Design review of the part built by this model. Coordinates are the model's own, in mm. Face numbers are marked on the shaded views. Coordinates: 2 decimals unless noted, no trailing zeros. Loops run counter-clockwise (first coordinate to the right, second up) from the corner with the lowest first, then second, coordinate; pieces in that order, holes last. Notation, with made-up numbers: M 56.25,8 L 91.25,8 A25 cw 91.25,43 Z; hole C 18.25,60.5 d5. An arc over 180 degrees is marked long. One line per item, written item: value.
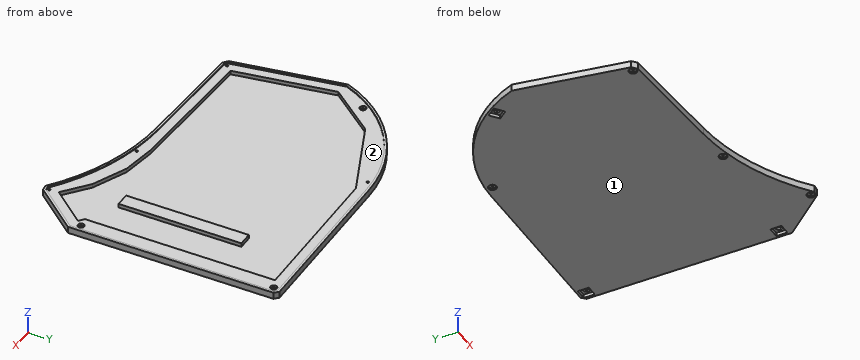
```python
from build123d import *

# Parameters (mm, degrees)
PAD001_DEPTH         = 3.4
POCKET006_DEPTH      = 0.4
SKETCH011_R          = 1.6
SKETCH011_W          = 7
SKETCH011_H          = 62
POCKET007_DEPTH      = 2
SKETCH012_W          = 5.6
SKETCH012_H          = 5.6
POCKET008_DEPTH      = 1.8
SKETCH014_R          = 0.6
POCKET010_DEPTH      = 0.001
POCKET010_DEPTH_BACK = 3.401
SKETCH016_R          = 2
POCKET012_DEPTH      = 1


with BuildPart() as part:
    # Sketch009 → Pad001 (new body)
    with BuildSketch(Plane(origin=(-70.9, 59.5, 0), x_dir=(1, 0, 0), z_dir=(0, 0, 1))):
        with BuildLine():
            ThreePointArc((129.954505, -55.0425), (90.803609, -67.301419), (65.635795, -99.699797))
            Line((65.635795, -99.699797), (75.365663, -154.835718))
            Line((75.365663, -154.835718), (77.709881, -156.921033))
            Line((77.709881, -156.921033), (133.968943, -160.182427))
            ThreePointArc((195.00443, -183.822904), (166.343475, -167.208769), (133.968943, -160.182427))
            Line((195.00443, -183.822904), (197.834526, -183.566965))
            Line((197.834526, -183.566965), (216.95, -160.867339))
            Line((216.95, -160.867339), (216.95, -57.0425))
            Line((214.95, -55.0425), (216.95, -57.0425))
            Line((214.95, -55.0425), (129.954505, -55.0425))
        make_face()
    extrude(amount=PAD001_DEPTH)

    # Sketch010 → Pocket006 (cut)
    with BuildSketch(Plane(origin=(-70.9, 59.5, 3.4), x_dir=(1, 0, 0), z_dir=(0, 0, 1))):
        with BuildLine():
            ThreePointArc((129.954505, -56.2425), (91.621754, -68.194493), (66.874586, -99.814544))
            Line((66.874586, -99.814544), (76.474909, -154.216377))
            Line((76.474909, -154.216377), (78.195777, -155.747186))
            Line((78.195777, -155.747186), (134.038391, -158.984439))
            ThreePointArc((195.379997, -182.584043), (166.5491, -166.00184), (134.038391, -158.984439))
            Line((195.379997, -182.584043), (197.234685, -182.416314))
            Line((197.234685, -182.416314), (215.75, -160.429378))
            Line((215.75, -160.429378), (215.75, -57.539556))
            Line((215.75, -57.539556), (214.452944, -56.2425))
            Line((214.452944, -56.2425), (129.954505, -56.2425))
        make_face()
    extrude(amount=-POCKET006_DEPTH, mode=Mode.SUBTRACT)

    # Sketch011 → Pocket007 (cut)
    with BuildSketch(Plane(origin=(-70.9, 59.5, 3), x_dir=(1, 0, 0), z_dir=(0, 0, 1))):
        with Locations((212.95, -59.0425)):
            Circle(SKETCH011_R)
        with Locations((212.95, -156.302532)):
            Circle(SKETCH011_R)
        with Locations((77.4441, -85.981596)):
            Circle(SKETCH011_R)
        Polygon((72.012841, -101.311041), (90.572874, -77.866788), (131.149099, -61.0425), (207.95, -61.0425), (207.95, -87.0425), (207.95, -156.967837), (210.542474, -159.161469), (195.830749, -176.631643), (183.495202, -166.193872), (166.255124, -158.080894), (149.066225, -155.047559), (80.797353, -151.089943), align=None)
        with Locations((187.45, -118.0425)):
            Rectangle(SKETCH011_W, SKETCH011_H, mode=Mode.SUBTRACT)
    extrude(amount=-POCKET007_DEPTH, mode=Mode.SUBTRACT)

    # Sketch012 → Pocket008 (cut)
    with BuildSketch(Plane(origin=(-70.9, 59.5, 0), x_dir=(1, 0, 0), z_dir=(0, 0, 1))):
        Polygon((81.377006, -85.514821), (76.978793, -82.04845), (73.512422, -86.446662), (77.910635, -89.913033), align=None)
        with Locations((212.95, -59.0425)):
            Rectangle(SKETCH012_W, SKETCH012_H)
        with Locations((212.95, -156.302532)):
            Rectangle(SKETCH012_W, SKETCH012_H)
    extrude(amount=POCKET008_DEPTH, mode=Mode.SUBTRACT)

    # Sketch014 → Pocket010 (cut, two sides)
    with BuildSketch(Plane(origin=(-70.9, 59.5, 0), x_dir=(1, 0, 0), z_dir=(0, 0, 1))) as pocket010_sk:
        with Locations((78.157217, -154.251862)):
            Circle(SKETCH014_R)
        with Locations((152.755217, -160.120567)):
            Circle(SKETCH014_R)
        with Locations((124.670042, -58.583126)):
            Circle(SKETCH014_R)
        with Locations((196.202376, -181.31749)):
            Circle(SKETCH014_R)
    extrude(amount=-POCKET010_DEPTH, mode=Mode.SUBTRACT)
    extrude(pocket010_sk.sketch, amount=POCKET010_DEPTH_BACK, mode=Mode.SUBTRACT)

    # Sketch016 → Pocket012 (cut)
    with BuildSketch(Plane(origin=(-70.9, 59.5, 0), x_dir=(1, 0, 0), z_dir=(0, 0, 1))):
        with Locations((78.157217, -154.251862)):
            Circle(SKETCH016_R)
        with Locations((152.755217, -160.120567)):
            Circle(SKETCH016_R)
        with Locations((124.670042, -58.583126)):
            Circle(SKETCH016_R)
        with Locations((196.202376, -181.31749)):
            Circle(SKETCH016_R)
    extrude(amount=POCKET012_DEPTH, mode=Mode.SUBTRACT)


with BuildPart() as part_1:
    # Body001 placement: moved
    add(part.part.moved(Location((0, 0, -3))))


solid = part_1.part
```
(1) We need section B-B on x = 14. State the section outline as (y, z) points, then the cut area to 3 significant figures.
Reply:
outline: M -97.84,-3 L -12.4,-3 L -12.4,0.4 L -14,0.4 L -14,0 L -25.53,0 L -25.53,-2 L -91.83,-2 L -91.83,0 L -96.64,0 L -96.64,0.4 L -97.84,0.4 Z
area: 125 mm2
(2) To check wall thickness, follow line 1 along X through (y, z) = (-86.5, -1.95); line 2 along Y through (x, z) = (142.05, -0.9); line 3 along X through (y, z) = (-52.5, -1.2). State the ranges of each line that lie inside material, in increasing order. Write a range as [from, to].
Reply:
line 1: x = [2.91, 9], [113.05, 120.05], [137.05, 146.05]
line 2: y = [-106.12, -98.4], [-95.2, -1.14], [2.06, 4.46]
line 3: x = [-3.09, 3], [113.05, 120.05], [137.05, 146.05]
(3) Mouldability with a two-part tool opening along Y and no side actions: class the marked faces 1 and 2 as released by +Y, released by -Y, zero draft, split by the parting line, or undercut.
Reply:
face 1: zero draft
face 2: undercut
(4) We need section A-A on y = -37. State the section outline as (x, z) points.
Reply:
outline: M -3.98,-3 L 146.05,-3 L 146.05,0.4 L 144.85,0.4 L 144.85,0 L 137.05,0 L 137.05,-2 L 120.05,-2 L 120.05,0 L 113.05,0 L 113.05,-2 L 4.92,-2 L 4.92,0 L -2.67,0 L -2.67,0.4 L -3.98,0.4 Z
(5) Insertion check: pin 1 (2 mm diameter, centred on x = 125, y = -121, fed in from -Z); pin 2 (1 mm diameter, centred on x = 73, y = -33, fed in from +Z); pin 3 (1 mm diameter, centred on y = -45.5, z = -1, fed in from -X); pin 4 (1.1 mm diameter, centred on x = 53.77, y = 0.92, fed in from -Z). Each pin has a flat end and moves straight along its axis. Give the tip position at first contact, or say it passes through.
Reply:
pin 1: stops at z = -2
pin 2: stops at z = -2
pin 3: stops at x = -4.42
pin 4: passes through
(6) We need section C-C on y = -79.5. State the section outline as (x, z) points.
Reply:
outline: M 1.67,-3 L 146.05,-3 L 146.05,0.4 L 144.85,0.4 L 144.85,0 L 137.05,0 L 137.05,-2 L 120.05,-2 L 120.05,0 L 113.05,0 L 113.05,-2 L 7.76,-2 L 7.76,0 L 2.89,0 L 2.89,0.4 L 1.67,0.4 Z
